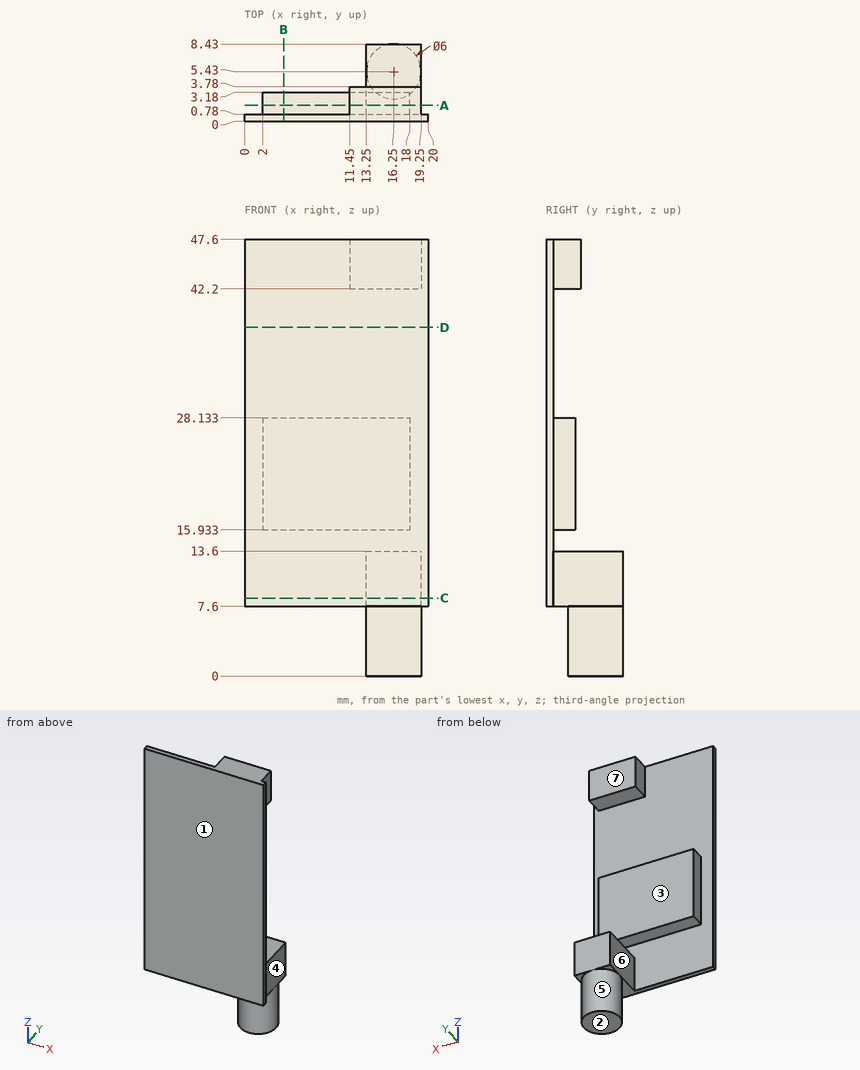
Verification items for this drawing (mm, ordinates from the low corner). A direction names the side the tool comes from. Coordinates: 2 decimals unless noted, no trailing zeros. Write each loop counter-clockwise with the first axis right and the second up, starting at its lowest first coordinate (ties: lowest second). Pieces come first, ordered by that corner, then holes. Notation, with made-up numbers: M -3,79 L 38,79 A17 ccw 38,86 Z; hole C 13,68 d6. An arc over 180 degrees is marked long. Answer as a JSON object with one key per item and string values. Group by question number.
(1) Material ranges on line 1 (Z direction, x = 9.5, y = 1); line 2 (Y direction, x = 7.75, z = 43); line 3 (Z direction, x = 15.75, y = 7), recorded low to high.
(2) Cross-section at D-D, the plane z = 38. Record the cut outline in (x, y), and give its area (3 significant figures).
(3) Cross-section at A-A, the plane y = 1.75. Record the cut outline in (x, z).
(4) Tool access check on the marked faces 4, 5, 6 and 7. Record the directions out of +Z, -Z, +X, -X, +Y, -Y that give a thin tool (end or side, any length) a straight path to the whole face; none if there is none.
(5) Cross-section at B-B, the plane x = 4.25. Record the cut outline in (y, z).
(6) Release check for a two-part mould opening along Z. For the marked faces 1, 2 and 3 record: +Z half, -Z half, draft (parallel to the pull), parting line (faces both ways), or undercut.
(7) Gauge pin test, flat ends, axial feed: pin 1 (0.9 mm diameter, centred on y = 1.5, z = 44.5, fed in from -X); pin 2 (4 mm diameter, centred on y = 3.5, z = 18.5, fed in from +X); pin 3 (10 mm diameter, centred on x = 13.5, z = 21, fed in from +Y); pin 4 (1 mm diameter, centred on x = 7, y = 5.5, fed in from -Z). Record the tip position at first contact, or that the pin passes through.
(8) Cross-section at C-C, the plane z = 8.5. Record the cut outline in (x, y), and give its area (3 significant figures).
Reply:
{
 "1": {"line 1": "15.93 to 28.13", "line 2": "0 to 0.78", "line 3": "0 to 13.6"},
 "2": {"outline": "M 0,0 L 20,0 L 20,0.78 L 0,0.78 Z", "area": "15.6 mm²"},
 "3": {"outline": "M 2,15.93 L 18,15.93 L 18,28.13 L 2,28.13 Z; M 11.45,42.2 L 19.25,42.2 L 19.25,47.6 L 11.45,47.6 Z; M 13.25,7.6 L 19.25,7.6 L 19.25,13.6 L 13.25,13.6 Z"},
 "4": {"face 4": "+Z, -Z, +X, +Y", "face 5": "-Z", "face 6": "-Z, -X, +Y", "face 7": "+Z, +X, -X, +Y"},
 "5": {"outline": "M 0,7.6 L 0.78,7.6 L 0.78,15.93 L 3.18,15.93 L 3.18,28.13 L 0.78,28.13 L 0.78,47.6 L 0,47.6 Z"},
 "6": {"face 1": "draft", "face 2": "-Z half", "face 3": "undercut"},
 "7": {"pin 1": "x = 11.45", "pin 2": "x = 18", "pin 3": "y = 3.18", "pin 4": "through"},
 "8": {"outline": "M 0,0 L 20,0 L 20,0.78 L 19.25,0.78 L 19.25,8.43 L 13.25,8.43 L 13.25,0.78 L 0,0.78 Z", "area": "61.5 mm²"}
}
